Design review of the part shown in the three views and the two pictorial views. Dimensions are in mm from the part's minimum x, y and z. Coordinates: 2 decimals unless noted, no trailing zeros. Order: outer loops, then holes, each group sorted by start corner. A loop starts at its lowest first (then second) coordinate and runs counter-clockwise, first axis right, second up. Notation, with made-up numbers: M 68.5,30.5 L 74.5,30.5 A18 cw 74.5,37.5 Z; hole C 88.5,37 d4. An arc over 180 degrees is marked long. Use CSV: the item, a comma, the result in double quotes.
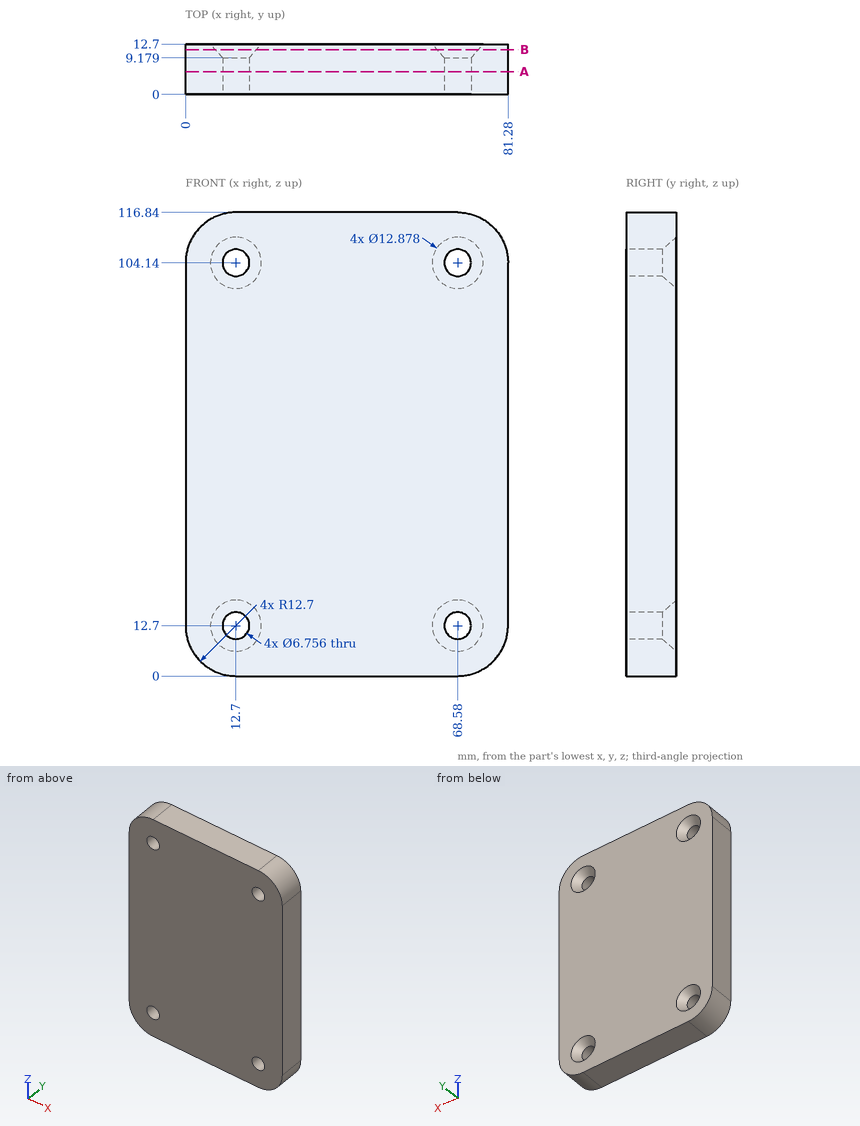
(1) Add section A-A on y = 5.75. State the section outline as (x, z) points.
The answers:
outline,"M 0,12.7 A12.7 ccw 12.7,0 L 68.58,0 A12.7 ccw 81.28,12.7 L 81.28,104.14 A12.7 ccw 68.58,116.84 L 12.7,116.84 A12.7 ccw 0,104.14 Z; hole C 12.7,12.7 d6.76; hole C 12.7,104.14 d6.76; hole C 68.58,12.7 d6.76; hole C 68.58,104.14 d6.76"
(2) Clearance check with flat-ended pins moving along their axes: P1, Ø5.5, axis at x = 68.58, z = 12.7, coming from the -Y side; P2, Ø1, axis at x = 70.5, y = 9, coming from the -Z side. State where each tip first meets the part, or that it passes through.
The answers:
P1,"passes through"
P2,"stops at z = 0.08"
(3) Add section B-B on y = 11.25. State the section outline as (x, z) points.
The answers:
outline,"M 0,12.7 A12.7 ccw 12.7,0 L 68.58,0 A12.7 ccw 81.28,12.7 L 81.28,104.14 A12.7 ccw 68.58,116.84 L 12.7,116.84 A12.7 ccw 0,104.14 Z; hole C 12.7,12.7 d10.36; hole C 12.7,104.14 d10.36; hole C 68.58,12.7 d10.36; hole C 68.58,104.14 d10.36"
(4) Wall thickness on probe 1 along Z at (x, y) = (68.58, 4.5); probe 2 along X at (y, z) = (3.25, 104.14); probe 3 along Z at (x, y) = (67, 5.5) (1 decimal): over which ranges is each line inside the solid? List them lowest first.
The answers:
probe 1,"z = 0 to 9.32, 16.08 to 100.76, 107.52 to 116.84"
probe 2,"x = 0 to 9.32, 16.08 to 65.2, 71.96 to 81.28"
probe 3,"z = 0 to 9.7, 15.7 to 101.2, 107.1 to 116.8"
